Check sheet for the modelled part. Datum: model origin and axes. Units: mm. Face numbers are marked on the shaded views. A direction names the side the tool comes from. Coordinates: 2 decimals unless noted, no trailing zeros. Order: outer loops, then holes, each group sorted by start corner. A loop starts at its lowest first (then second) coordinate and runs counter-clockwise, first axis right, second up.
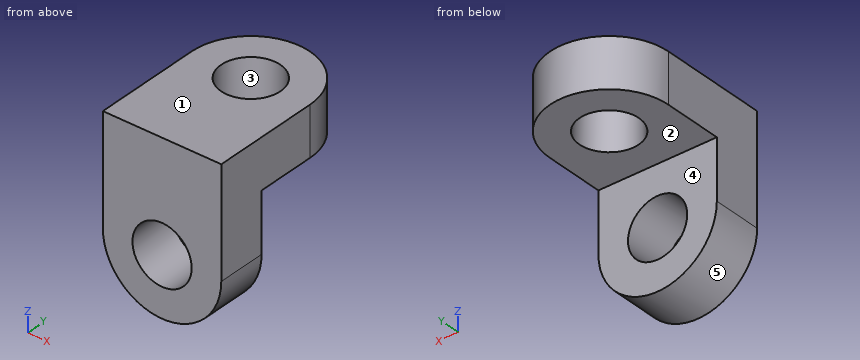
from build123d import *

# Parameters (mm, degrees)
SKETCH1_R           = 6
BOSS_EXTRUDE1_DEPTH = 10
BOSS_EXTRUDE2_DEPTH = 24


with BuildPart() as part:
    # Sketch1 → Boss-Extrude1 (new body)
    with BuildSketch(Plane.XY):
        with BuildLine():
            Line((12, 0), (12, -12))
            Line((12, -12), (-12, -12))
            Line((-12, -12), (-12, 0))
            ThreePointArc((-12, 0), (0, 12), (12, 0))
        make_face()
        Circle(SKETCH1_R, mode=Mode.SUBTRACT)
    extrude(amount=BOSS_EXTRUDE1_DEPTH)

    # Sketch3 → Boss-Extrude2 (add)
    with BuildSketch(Plane.ZY.offset(12)):
        Polygon((0, -12), (10, -22), (10, -12), align=None)
    extrude(amount=-BOSS_EXTRUDE2_DEPTH)

    # Mirror6: part across plane


with BuildPart() as part_1:
    add(part.part)
    add(part.part.mirror(Plane(origin=(26.142135624, -12, 0), x_dir=(0, -0.7071067811865439, 0.7071067811865512), z_dir=(0, -0.7071067811865513, -0.7071067811865438))))


solid = part_1.part
(1) Cross-section at B-B (y = -16). Enter the section's corners in (x, z), and give its area (3 significant figures).
Filled in:
outline: (-12, -12) arc R12 ccw to (12, -12) - (12, 10) - (-12, 10) - close; hole circle Ø12 at (0, -12)
area: 641 mm2
(2) Cross-section at A-A (x = 0). Enter the section's corners in (y, z).
Filled in:
outline: (-22, -24) - (-12, -24) - (-12, -18) - (-22, -18) - close; (-22, -6) - (-12, -6) - (-12, 0) - (-6, 0) - (-6, 10) - (-22, 10) - close; (6, 0) - (12, 0) - (12, 10) - (6, 10) - close
(3) Release check for a two-part mould opening along Y. For the marked faces 3, 4 and 5 record: +Y half, -Y half, draft (parallel to the pull), parting line (faces both ways), or undercut.
Filled in:
face 3: undercut
face 4: +Y half
face 5: draft
(4) Cross-section at D-D (y = -3). Enter the section's corners in (x, z).
Filled in:
outline: (-12, 0) - (-5.2, 0) - (-5.2, 10) - (-12, 10) - close; (5.2, 0) - (12, 0) - (12, 10) - (5.2, 10) - close
(5) Cross-section at C-C (z = 1.5). Enter the section's corners in (x, y).
Filled in:
outline: (-12, -22) - (12, -22) - (12, 0) arc R12 ccw to (-12, 0) - close; hole circle Ø12 at (0, 0)
(6) Go/stop test with flat-tipped pins: P1, Ø7, axis at x = -3.5, z = -9.5, coming from the +Y side; P2, Ø9.5, axis at x = 0, y = 0, coming from the +Z side. Record where each tip stops, or that it passes through.
Filled in:
P1: stops at y = -12
P2: passes through
(7) Thickness scan on probe 1 along X at (y, z) = (-19.25, -12); probe 2 along Y at (x, z) = (0, 8); probe 3 along Y at (x, z) = (8, -2). Record the ranges inside material, lowest first.
Filled in:
probe 1: x = -12 to -6, 6 to 12
probe 2: y = -22 to -6, 6 to 12
probe 3: y = -22 to -12
(8) Tool access check on the marked faces 1 and 2. Record the directions out of +Z, -Z, +X, -X, +Y, -Y that give a thin tool (end or side, any length) a straight path to the whole face; none if there is none.
Filled in:
face 1: +Z, +X, -X, +Y, -Y
face 2: -Z, +X, -X, +Y
